from build123d import *

# Parameters (mm, degrees)
BASE_FLANGE1_DEPTH           = 115.57
EDGE_FLANGE1_DEPTH           = 115.57
EDGE_FLANGE2_STRIP_CUT_DEPTH = 115.57
EDGE_FLANGE2_DEPTH           = 115.57
EDGE_FLANGE3_DEPTH           = 115.57
SKETCH20_R                   = 6.35
CUT_EXTRUDE1_DEPTH           = 2.65684


# Sheet-metal steps are written as plain solids
with BuildPart() as part:
    # Sketch1 → Base-Flange1 (new body)
    with BuildSketch(Plane.XY):
        with BuildLine():
            ThreePointArc((-50.8, 170.388379885), (-140.856418383, 108.500273734), (-177.710803869, 5.63118))
            Line((-177.710803869, 5.63118), (-180.366311024, 5.715325918))
            ThreePointArc((-180.366311024, 5.715325918), (-142.961215721, 110.121577824), (-51.559097143, 172.934469105))
            Line((-51.559097143, 172.934469105), (-50.8, 170.388379885))
        make_face()
    extrude(amount=BASE_FLANGE1_DEPTH)

    # Edge-Flange1 section (across the edge) → Edge-Flange1 (add)
    with BuildSketch(Plane(origin=(-49.291175996, 173.610632552, 115.57), x_dir=(-0.9999999996342678, -2.7045604981235094e-05, 0), z_dir=(0, 0, -1))):
        with BuildLine():
            Line((-2.65684, 2.366572064), (-2.65684, 76.2))
            Line((-2.65684, 76.2), (0, 76.2))
            Line((0, 76.2), (0, 2.366572064))
            ThreePointArc((0, 2.366572064), (0.62936233, 0.469112223), (2.267939433, -0.676102109))
            Line((2.267939433, -0.676102109), (1.508911151, -3.222211858))
            ThreePointArc((1.508911151, -3.222211858), (-1.500827273, -1.118682173), (-2.65684, 2.366572064))
        make_face()
    extrude(amount=EDGE_FLANGE1_DEPTH)

    # Edge-Flange2 strip (across the edge) → Edge-Flange2 strip cut (cut)
    with BuildSketch(Plane(origin=(-49.293236871, 249.810632524, 115.57), x_dir=(-0.766027058259036, -0.6428083275868535, 0), z_dir=(0, 0, -1))):
        Polygon((-12.205285278, 10.412383287), (-1.292448625, -2.593029), (0.742808893, -0.885245167), (-10.17002776, 12.12016712), align=None)
    extrude(amount=EDGE_FLANGE2_STRIP_CUT_DEPTH, mode=Mode.SUBTRACT)

    # Edge-Flange2 section (across the edge) → Edge-Flange2 (add)
    with BuildSketch(Plane(origin=(-49.293236871, 249.810632524, 115.57), x_dir=(-0.766027058259036, -0.6428083275868535, 0), z_dir=(0, 0, -1))):
        with BuildLine():
            Line((-2.65684, 1.155605494), (-2.65684, 101.6))
            Line((-2.65684, 101.6), (0, 101.6))
            Line((0, 101.6), (0, 1.155605494))
            ThreePointArc((0, 1.155605494), (0.191475929, 0.069691539), (0.742808893, -0.885245167))
            Line((0.742808893, -0.885245167), (-1.292448625, -2.593029))
            ThreePointArc((-1.292448625, -2.593029), (-2.305137014, -0.839001259), (-2.65684, 1.155605494))
        make_face()
    extrude(amount=EDGE_FLANGE2_DEPTH)

    # Edge-Flange3 section (across the edge) → Edge-Flange3 (add)
    with BuildSketch(Plane(origin=(-180.463740314, 2.640617339, 0), x_dir=(8.626632785422443e-05, 0.9999999962790604, 0), z_dir=(0, 0, 1))):
        with BuildLine():
            Line((-2.65684, 3.076251829), (-2.65684, 57.15))
            Line((-2.65684, 57.15), (0, 57.15))
            Line((0, 57.15), (0, 3.076251829))
            ThreePointArc((0, 3.076251829), (0.894756196, 0.86692768), (3.074716973, -0.097164046))
            Line((3.074716973, -0.097164046), (2.990800136, -2.75267845))
            ThreePointArc((2.990800136, -2.75267845), (-1.013351819, -0.981834768), (-2.65684, 3.076251829))
        make_face()
    extrude(amount=EDGE_FLANGE3_DEPTH)

    # Sketch20 → Cut-Extrude1 (cut)
    with BuildSketch(Plane(origin=(0.000226453, 2.625049375, 0), x_dir=(0.9999999962790604, -8.626632785420363e-05, 0), z_dir=(8.626632785420363e-05, 0.9999999962790604, 0))):
        with Locations(Location((-218.563967439, -31.75, 0), (0, 0, 180))):
            Circle(SKETCH20_R)
        with Locations(Location((-218.563967439, -82.55, 0), (0, 0, 180))):
            Circle(SKETCH20_R)
    extrude(amount=-CUT_EXTRUDE1_DEPTH, mode=Mode.SUBTRACT)


solid = part.part
Here's how the part is built. I have some questions about the finished solid (model axes, mm). Coordinates: 2 decimals unless noted, no trailing zeros. Order: outer loops, then holes, each group sorted by start corner. A loop starts at its lowest first (then second) coordinate and runs counter-clockwise, first axis right, second up. Notation, with made-up numbers: (-16.75, 57) - (0.25, 57) arc R20 ccw to (0.25, 93) - close; hole circle Ø3 at (26.25, -34.5). An arc over 180 degrees is marked (long way). Use CSV: the item, a comma, the result in double quotes. Start each with the question number.
1. Suppose I cut it at B-B on x = -88. List the corners of the cut face in (y, z) for me.
2. Suppose I cut it at A-A on z = 20.5. List the corners of the cut face in (x, y) for me (3 decimals), then the cut area to 3 significant figures.
3. Suppose I cut it at D-D on y = 268.5. List the corners of the cut face in (x, z) for me.
4. I'm going to push flat-ended pins straight in: pin 1 (20.5 mm diameter, centred on x = -218.56, z = 82.55, fed in from +Y); pin 2 (2 mm diameter, centred on x = -159, z = 67, fed in from -Y); pin 3 (3 mm diameter, centred on y = 293, z = 16.5, fed in from -X). Where does each tip first touch, or does it pass through?
5. Suppose I cut it at C-C on x = -134. List the corners of the cut face in (y, z) for me.
6. Please list where these lines run through material, in increasing order: line 1 (X direction, y = 244.5, z = 98.5); line 2 (Y direction, x = -103, z = 38.5); line 3 (Y direction, x = -95, z = 27). Write a range as from..to.
7. If we mould it in two halves opening along X, with no side actions, what happens to faces 1 (the face through (-143.919, 108.867, 56.976)), 2 (the face through (-213.88, 1.33, 86.84)), 3 (the face through (-79.8, 290.3, 58.6))? For each: +X half, -X half, draft (parallel to the pull), parting line (faces both ways), or undercut.
Output:
1,outline,"(154.5, 0) - (157.55, 0) - (157.55, 115.57) - (154.5, 115.57) - close; (295.94, 0) - (300.07, 0) - (300.07, 115.57) - (295.94, 115.57) - close"
2,outline,"(-237.614, -0.011) - (-183.54, -0.016) arc R5.832 ccw to (-177.711, 5.631) arc R177.8 cw to (-50.8, 170.388) arc R5.832 ccw to (-46.634, 175.977) - (-46.636, 248.655) arc R5.832 ccw to (-48.001, 252.404) - (-112.567, 329.347) - (-114.603, 327.639) - (-50.036, 250.696) arc R3.175 cw to (-49.293, 248.655) - (-49.291, 175.977) arc R3.175 cw to (-51.559, 172.934) arc R180.457 ccw to (-180.366, 5.715) arc R3.175 cw to (-183.54, 2.641) - (-237.614, 2.646) - close"
2,area,"1,240 mm2"
3,outline,"(-64.98, 0) - (-61.51, 0) - (-61.51, 115.57) - (-64.98, 115.57) - close"
4,pin 1,"stops at y = 2.64"
4,pin 2,"stops at y = 77.54"
4,pin 3,"stops at x = -86.79"
5,outline,"(116.86, 0) - (120.87, 0) - (120.87, 115.57) - (116.86, 115.57) - close"
6,line 1,"x = -49.29..-46.64"
6,line 2,"y = 144.93..148.17, 313.81..317.95"
6,line 3,"y = 150.29..153.43, 304.28..308.41"
7,face 1,"-X half"
7,face 2,"undercut"
7,face 3,"+X half"
